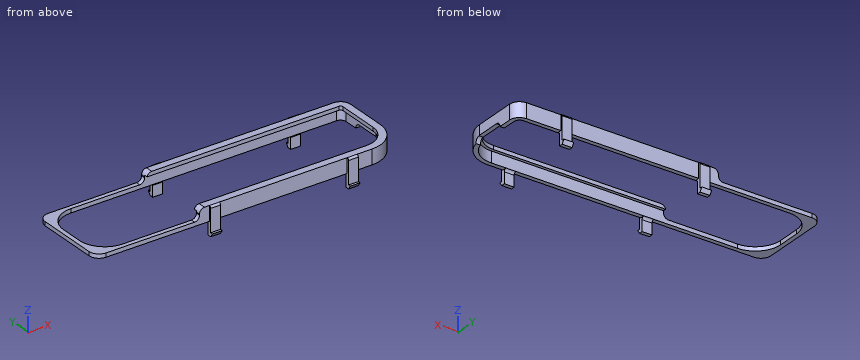
```python
from build123d import *

# Parameters (mm, degrees)
BOSS_EXTRUDE2_THICKNESS_OF_TC_PCB_DEPTH = 4.5
BOSS_EXTRUDE3_RETAINING_TOP_DEPTH       = 1.5
CUT_EXTRUDE1_START                      = -2.881
CUT_EXTRUDE1_EXPOSED_TC_FRONT_DEPTH     = 2.881
FILLET1_R                               = 2
SKETCH7_W                               = 2
SKETCH7_H                               = 14
CUT_EXTRUDE1_USBC_CUTOUT_DEPTH          = 5
FILLET3_R                               = 2
SKETCH8_W                               = 4
SKETCH8_H                               = 1.5
BOSS_EXTRUDE5_SNAP_POSTS_DEPTH          = 5.5
BOSS_EXTRUDE6_SNAP_NOTCH_1_DEPTH        = 4
BOSS_EXTRUDE7_SNAP_NOTCH_2_DEPTH        = 4
SKETCH11_W                              = 4
SKETCH11_H                              = 2.5
BOSS_EXTRUDE1_SNAP_BUMPS_DEPTH          = 6
FILLET6_R                               = 1
FILLET7_R                               = 0.75
BOSS_EXTRUDE1_START                     = -1.619
BOSS_EXTRUDE1_DEPTH                     = 1.619
FILLET8_R                               = 4


with BuildPart() as part:
    # Sketch3 → Boss-Extrude2 - thickness of TC + PCB (new body)
    with BuildSketch(Plane.XY):
        with BuildLine():
            Line((122, -4.5), (122, 12.5))
            ThreePointArc((122, 12.5), (120.828427125, 15.328427125), (118, 16.5))
            Line((118, 16.5), (10, 16.5))
            ThreePointArc((10, 16.5), (1.514718626, 12.985281374), (-2, 4.5))
            Line((-2, 4.5), (-2, -4.5))
            ThreePointArc((-2, -4.5), (1.514718626, -12.985281374), (10, -16.5))
            Line((10, -16.5), (110, -16.5))
            ThreePointArc((110, -16.5), (118.485281374, -12.985281374), (122, -4.5))
        make_face()
        with BuildLine():
            Line((118, 14.75), (10, 14.75))
            ThreePointArc((10, 14.75), (2.752155493, 11.747844507), (-0.25, 4.5))
            Line((-0.25, 4.5), (-0.25, -4.5))
            ThreePointArc((-0.25, -4.5), (2.752155493, -11.747844507), (10, -14.75))
            Line((10, -14.75), (110, -14.75))
            ThreePointArc((110, -14.75), (117.247844507, -11.747844507), (120.25, -4.5))
            Line((120.25, -4.5), (120.25, 12.5))
            ThreePointArc((120.25, 12.5), (119.590990258, 14.090990258), (118, 14.75))
        make_face(mode=Mode.SUBTRACT)
    extrude(amount=BOSS_EXTRUDE2_THICKNESS_OF_TC_PCB_DEPTH)

    # Sketch4 → Boss-Extrude3 - retaining top (add)
    with BuildSketch(Plane.XY.offset(4.5)):
        with BuildLine():
            Line((40, 13.5), (118, 13.5))
            ThreePointArc((118, 13.5), (118.707106781, 13.207106781), (119, 12.5))
            Line((119, 12.5), (119, -4.5))
            ThreePointArc((119, -4.5), (116.363961031, -10.863961031), (110, -13.5))
            Line((110, -13.5), (40, -13.5))
            Line((40, -13.5), (40, -16.5))
            Line((40, -16.5), (110, -16.5))
            ThreePointArc((110, -16.5), (118.485281374, -12.985281374), (122, -4.5))
            Line((122, -4.5), (122, 12.5))
            ThreePointArc((122, 12.5), (120.828427125, 15.328427125), (118, 16.5))
            Line((118, 16.5), (40, 16.5))
            Line((40, 16.5), (40, 13.5))
        make_face()
    extrude(amount=BOSS_EXTRUDE3_RETAINING_TOP_DEPTH)

    # Sketch5 → Cut-Extrude1 - exposed TC front (cut)
    with BuildSketch(Plane.XY.offset(4.5).offset(CUT_EXTRUDE1_START)):
        with BuildLine():
            Line((40, -16.5), (40, -14.75))
            Line((40, -14.75), (10, -14.75))
            ThreePointArc((10, -14.75), (2.752155493, -11.747844507), (-0.25, -4.5))
            Line((-0.25, -4.5), (-0.25, 4.5))
            ThreePointArc((-0.25, 4.5), (2.752155493, 11.747844507), (10, 14.75))
            Line((10, 14.75), (40, 14.75))
            Line((40, 14.75), (40, 16.5))
            Line((40, 16.5), (10, 16.5))
            ThreePointArc((10, 16.5), (1.514718626, 12.985281374), (-2, 4.5))
            Line((-2, 4.5), (-2, -4.5))
            ThreePointArc((-2, -4.5), (1.514718626, -12.985281374), (10, -16.5))
            Line((10, -16.5), (40, -16.5))
        make_face()
    extrude(amount=CUT_EXTRUDE1_EXPOSED_TC_FRONT_DEPTH, mode=Mode.SUBTRACT)

    # Fillet1
    fillet1_edges = [part.edges().sort_by_distance(p)[0] for p in [
        (40, 15, 6),
        (40, 15.625, 1.619),
        (40, -15, 6),
        (40, -15.625, 1.619),
    ]]
    fillet(fillet1_edges, radius=FILLET1_R)

    # Sketch7 → Cut-Extrude1 - USBC cutout (cut)
    with BuildSketch(Plane(origin=(122, 0, 0), x_dir=(0, 0, -1), z_dir=(1, 0, 0))):
        with Locations((-1, 0)):
            Rectangle(SKETCH7_W, SKETCH7_H)
    extrude(amount=-CUT_EXTRUDE1_USBC_CUTOUT_DEPTH, mode=Mode.SUBTRACT)

    # Fillet3
    fillet3_edges = [part.edges().sort_by_distance(p)[0] for p in [
        (121.125, 7, 2),
        (120.838571135, -7, 2),
    ]]
    fillet(fillet3_edges, radius=FILLET3_R - 0.0001)  # a hair under: the kernel refuses the full size

    # Sketch8 → Boss-Extrude5 - snap posts (add)
    with BuildSketch(Plane(origin=(0, 0, 0), x_dir=(-1, 0, 0), z_dir=(0, 0, -1))):
        with Locations((-46, -16.5)):
            Rectangle(SKETCH8_W, SKETCH8_H)
        with Locations((-102, -16.5)):
            Rectangle(SKETCH8_W, SKETCH8_H)
    boss_extrude5_snap_posts = extrude(amount=BOSS_EXTRUDE5_SNAP_POSTS_DEPTH)

    # Sketch9 → Boss-Extrude6 - snap notch 1 (add)
    with BuildSketch(Plane.ZY.offset(-44)):
        Polygon((-5.5, -17.25), (-4, -18.25), (-4, -17.25), align=None)
    boss_extrude6_snap_notch_1 = extrude(amount=-BOSS_EXTRUDE6_SNAP_NOTCH_1_DEPTH)

    # Sketch10 → Boss-Extrude7 - snap notch 2 (add)
    with BuildSketch(Plane.ZY.offset(-100)):
        Polygon((-4, -18.25), (-4, -17.25), (-5.5, -17.25), align=None)
    boss_extrude7_snap_notch_2 = extrude(amount=-BOSS_EXTRUDE7_SNAP_NOTCH_2_DEPTH)

    # Sketch11 → Boss-Extrude1 - snap bumps (add)
    with BuildSketch(Plane(origin=(0, 0, 0), x_dir=(-1, 0, 0), z_dir=(0, 0, -1))):
        with Locations((-46, -16)):
            Rectangle(SKETCH11_W, SKETCH11_H)
        with Locations((-102, -16)):
            Rectangle(SKETCH11_W, SKETCH11_H)
    boss_extrude1_snap_bumps = extrude(amount=-BOSS_EXTRUDE1_SNAP_BUMPS_DEPTH)

    # Mirror1: Boss-Extrude5 - snap posts, Boss-Extrude6 - snap notch 1, Boss-Extrude7 - snap notch 2, Boss-Extrude1 - snap bumps across plane
    add(boss_extrude5_snap_posts.mirror(Plane.ZX))
    add(boss_extrude6_snap_notch_1.mirror(Plane.ZX))
    add(boss_extrude7_snap_notch_2.mirror(Plane.ZX))
    add(boss_extrude1_snap_bumps.mirror(Plane.ZX))

    # Fillet6
    fillet6_edges = [part.edges().sort_by_distance(p)[0] for p in [
        (46, -15.75, 0),
        (102, -15.75, 0),
        (46, 15.75, 0),
        (102, 15.75, 0),
    ]]
    fillet(fillet6_edges, radius=FILLET6_R - 0.0001)  # a hair under: the kernel refuses the full size

    # Fillet7
    fillet7_edges = [part.edges().sort_by_distance(p)[0] for p in [
        (46, -17.25, 6),
        (102, -17.25, 6),
        (46, 17.25, 6),
        (102, 17.25, 6),
    ]]
    fillet(fillet7_edges, radius=FILLET7_R)

    # Sketch13 → Boss-Extrude1 (add)
    with BuildSketch(Plane.XY.offset(1.619).offset(BOSS_EXTRUDE1_START)):
        with BuildLine():
            Line((-2, 4.5), (-2, 16.5))
            Line((-2, 16.5), (10, 16.5))
            ThreePointArc((10, 16.5), (1.514718626, 12.985281374), (-2, 4.5))
        make_face()
        with BuildLine():
            Line((-2, -4.5), (-2, -16.5))
            Line((-2, -16.5), (10, -16.5))
            ThreePointArc((10, -16.5), (1.514718626, -12.985281374), (-2, -4.5))
        make_face()
    extrude(amount=BOSS_EXTRUDE1_DEPTH)

    # Fillet8
    fillet8_edges = [part.edges().sort_by_distance(p)[0] for p in [
        (-2, 16.5, 0.8095),
        (-2, -16.5, 0.8095),
    ]]
    fillet(fillet8_edges, radius=FILLET8_R)


solid = part.part
```
Could you check a few things on this model? Use its own coordinates, in mm. Round coordinates to 2 decimals unless told otherwise and drop trailing zeros. Loops run counter-clockwise (first coordinate to the right, second up) from the corner with the lowest first, then second, coordinate; pieces in that order, holes last. Notation, with made-up numbers: (60.25, 21) - (73.25, 21) arc R15 cw to (73.25, 38) - close; hole circle Ø5 at (-34, 36). An arc over 180 degrees is marked (long way). Answer in a Markdown table with one row per item. Add a question column.
(1) If we section it at B-B (x = 107): Please give me the cut outline in (y, z).
(2) If we section it at A-A (z = -2.25): Please give me the cut outline in (x, y).
(3) I need wall thicknesses on line 1 along Y through (x, z) = (64.5, 1.25); line 2 along Z through (x, y) = (58.5, -16); line 3 along X through (y, z) = (-1.5, 0.5). Which ranges of each line are inside material? Lowest first, please.
(4) I'm going to push flat-ended pins straight in: pin 1 (1.2 mm diameter, centred on x = 102.5, z = -3, fed in from -Y); pin 2 (4 mm diameter, centred on y = -15.5, z = 3, fed in from -X); pin 3 (1.7 mm diameter, centred on y = 16, z = -1, fed in from +X); pin 4 (3 mm diameter, centred on y = 14, z = 1.5, fed in from -X). Where does each tip first touch, or does it pass through?
(5) If we section it at C-C (x = 26): Please give me the cut outline in (y, z).
Model answer:
| question | item | result |
|---|---|---|
| 1 | outline | (-16.5, 0) - (-14.75, 0) - (-14.75, 4.5) - (-13.5, 4.5) - (-13.5, 6) - (-16.5, 6) - close; (13.5, 4.5) - (14.75, 4.5) - (14.75, 0) - (16.5, 0) - (16.5, 6) - (13.5, 6) - close |
| 2 | outline | (44, -17.25) - (48, -17.25) - (48, -15.75) - (44, -15.75) - close; (44, 15.75) - (48, 15.75) - (48, 17.25) - (44, 17.25) - close; (100, -17.25) - (104, -17.25) - (104, -15.75) - (100, -15.75) - close; (100, 15.75) - (104, 15.75) - (104, 17.25) - (100, 17.25) - close |
| 3 | line 1 | y = -16.5 to -14.75, 14.75 to 16.5 |
| 3 | line 2 | z = 0 to 6 |
| 3 | line 3 | x = -2 to -0.25 |
| 4 | pin 1 | stops at y = -17.25 |
| 4 | pin 2 | stops at x = -1.69 |
| 4 | pin 3 | stops at x = 104 |
| 4 | pin 4 | stops at x = -2 |
| 5 | outline | (-16.5, 0) - (-14.75, 0) - (-14.75, 1.62) - (-16.5, 1.62) - close; (14.75, 0) - (16.5, 0) - (16.5, 1.62) - (14.75, 1.62) - close |
